```python
from build123d import *

# Parameters (mm, degrees)
SKETCH1_R               = 250
SKETCH1_R_2             = 6
SKETCH1_R_3             = 40
BOSS_EXTRUDE1_DEPTH     = 10
CUT_EXTRUDE1_DEPTH      = 354.694783677
CUT_EXTRUDE1_DEPTH_BACK = 354.694783677
SKETCH2_R               = 3


with BuildPart() as part:
    # Sketch1 → Boss-Extrude1 (new body)
    with BuildSketch(Plane(origin=(0, 0, 0), x_dir=(0, 0, -1), z_dir=(1, 0, 0))):
        Circle(SKETCH1_R)
        Circle(SKETCH1_R_2, mode=Mode.SUBTRACT)
        with Locations((0, 175)):
            Circle(SKETCH1_R_3, mode=Mode.SUBTRACT)
        with Locations((151.554445662, 87.5)):
            Circle(SKETCH1_R_3, mode=Mode.SUBTRACT)
        with Locations((151.554445662, -87.5)):
            Circle(SKETCH1_R_3, mode=Mode.SUBTRACT)
        with Locations((0, -175)):
            Circle(SKETCH1_R_3, mode=Mode.SUBTRACT)
        with Locations((-151.554445662, -87.5)):
            Circle(SKETCH1_R_3, mode=Mode.SUBTRACT)
        with Locations((-151.554445662, 87.5)):
            Circle(SKETCH1_R_3, mode=Mode.SUBTRACT)
    extrude(amount=BOSS_EXTRUDE1_DEPTH)

    # Sketch2 → Cut-Extrude1 (cut, two sides: drawn at the far end of the back side and taken through both)
    with BuildSketch(Plane.ZY.offset(-CUT_EXTRUDE1_DEPTH_BACK)):
        with Locations((-34.248705894, 43.035173342)):
            Circle(SKETCH2_R)
        with Locations((34.248705894, -43.035173342)):
            Circle(SKETCH2_R)
        with BuildLine():
            Line((-40, 175), (-40, 246.779253585))
            ThreePointArc((-40, 246.779253585), (0, 250), (40, 246.779253585))
            Line((40, 246.779253585), (40, 175))
            ThreePointArc((40, 175), (0, 215), (-40, 175))
        make_face()
        with BuildLine():
            Line((131.554445662, 122.141016151), (193.717102732, 158.030642944))
            ThreePointArc((193.717102732, 158.030642944), (216.506350946, 125), (233.717102732, 88.748610641))
            Line((233.717102732, 88.748610641), (171.554445662, 52.858983849))
            ThreePointArc((171.554445662, 52.858983849), (186.195461814, 107.5), (131.554445662, 122.141016151))
        make_face()
        with BuildLine():
            Line((171.554445662, -52.858983849), (233.717102732, -88.748610641))
            ThreePointArc((233.717102732, -88.748610641), (216.506350946, -125), (193.717102732, -158.030642944))
            Line((193.717102732, -158.030642944), (131.554445662, -122.141016151))
            ThreePointArc((131.554445662, -122.141016151), (186.195461814, -107.5), (171.554445662, -52.858983849))
        make_face()
        with BuildLine():
            Line((40, -175), (40, -246.779253585))
            ThreePointArc((40, -246.779253585), (0, -250), (-40, -246.779253585))
            Line((-40, -246.779253585), (-40, -175))
            ThreePointArc((-40, -175), (0, -215), (40, -175))
        make_face()
        with BuildLine():
            Line((-131.554445662, -122.141016151), (-193.717102732, -158.030642944))
            ThreePointArc((-193.717102732, -158.030642944), (-216.506350946, -125), (-233.717102732, -88.748610641))
            Line((-233.717102732, -88.748610641), (-171.554445662, -52.858983849))
            ThreePointArc((-171.554445662, -52.858983849), (-186.195461814, -107.5), (-131.554445662, -122.141016151))
        make_face()
        with BuildLine():
            Line((-171.554445662, 52.858983849), (-233.717102732, 88.748610641))
            ThreePointArc((-233.717102732, 88.748610641), (-216.506350946, 125), (-193.717102732, 158.030642944))
            Line((-193.717102732, 158.030642944), (-131.554445662, 122.141016151))
            ThreePointArc((-131.554445662, 122.141016151), (-186.195461814, 107.5), (-171.554445662, 52.858983849))
        make_face()
    extrude(amount=CUT_EXTRUDE1_DEPTH + CUT_EXTRUDE1_DEPTH_BACK, mode=Mode.SUBTRACT)


solid = part.part
```
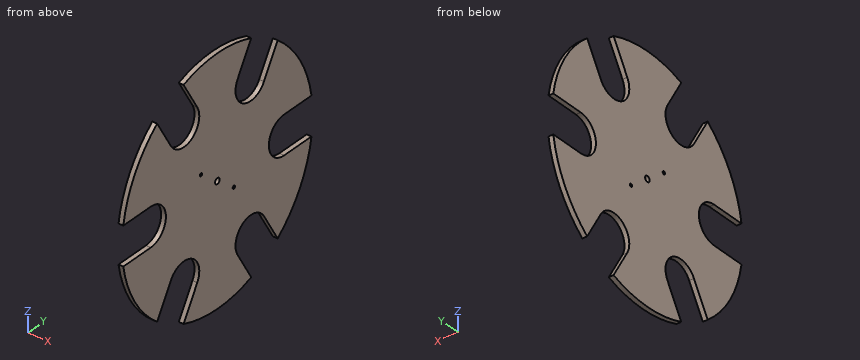
Part model, mm, in its own coordinate system. Round coordinates to 2 decimals unless told otherwise and drop trailing zeros. Loops run counter-clockwise (first coordinate to the right, second up) from the corner with the lowest first, then second, coordinate; pieces in that order, holes last. Notation, with made-up numbers: (18, 22.5) -> (31, 22.5) arc R8 cw to (31, 26.5) -> close; hole circle Ø6 at (72.5, 86). An arc over 180 degrees is marked (long way). Use a Markdown table: item, result.
1) Cut at D-D, the plane z = -101. List the corners of the cut face in (x, y).
The answers:
| item | result |
|---|---|
| outline | (0, -228.69) -> (10, -228.69) -> (10, 228.69) -> (0, 228.69) -> close |
2) Drop flat-ended pins along their axis: pin 1 Ø5 at (x, y) = (5.5, -222) entering from +Z; pin 2 Ø2 at (x, z) = (6, 97) entering from -Y; pin 3 Ø3 at (x, y) = (7, -218) entering from -Z. Give the stop position or say it passes through.
The answers:
| item | result |
|---|---|
| pin 1 | stops at z = 119.67 |
| pin 2 | stops at y = -230.83 |
| pin 3 | stops at z = -125.01 |
3) Cut at C-C, the plane x = 8.5. List the corners of the cut face in (y, z).
The answers:
| item | result |
|---|---|
| outline | (-246.78, -40) arc R250 ccw to (-158.03, -193.72) -> (-122.14, -131.55) arc R40 cw to (-52.86, -171.55) -> (-88.75, -233.72) arc R250 ccw to (88.75, -233.72) -> (52.86, -171.55) arc R40 cw to (122.14, -131.55) -> (158.03, -193.72) arc R250 ccw to (246.78, -40) -> (175, -40) arc R40 cw to (175, 40) -> (246.78, 40) arc R250 ccw to (158.03, 193.72) -> (122.14, 131.55) arc R40 cw to (52.86, 171.55) -> (88.75, 233.72) arc R250 ccw to (-88.75, 233.72) -> (-52.86, 171.55) arc R40 cw to (-122.14, 131.55) -> (-158.03, 193.72) arc R250 ccw to (-246.78, 40) -> (-175, 40) arc R40 cw to (-175, -40) -> close; hole circle Ø6 at (-43.04, 34.25); hole circle Ø12 at (0, 0); hole circle Ø6 at (43.04, -34.25) |
4) Probe line 1 (Y direction, x = 5.25, z = 133.5); line 2 (Y direction, x = 6.5, z = 120); line 3 (Z direction, x = 9.5, y = 61.5). List the from-to ranges inside material, lowest first. Write a range as [from, to].
The answers:
| item | result |
|---|---|
| line 1 | y = [-211.37, -123.26], [-51.81, 51.81], [123.26, 211.37] |
| line 2 | y = [-219.32, -112.08], [-62.92, 62.92], [112.08, 219.32] |
| line 3 | z = [-242.32, -186.52], [-121.16, 121.16], [186.52, 242.32] |
5) Cut at A-A, the plane y = 0. List the corners of the cut face in (x, z).
The answers:
| item | result |
|---|---|
| outline | (0, -250) -> (10, -250) -> (10, -6) -> (0, -6) -> close; (0, 6) -> (10, 6) -> (10, 250) -> (0, 250) -> close |
6) Cut at B-B, the plane z = 0. List the corners of the cut face in (x, y), and give its area (3 significant figures).
The answers:
| item | result |
|---|---|
| outline | (0, -135) -> (10, -135) -> (10, -6) -> (0, -6) -> close; (0, 6) -> (10, 6) -> (10, 135) -> (0, 135) -> close |
| area | 2,580 mm2 |
